Input: dimensioned drawing with shaded views. Units: mm. Origin: part minimum x, y, z. Round coordinates to 2 decimals unless told otherwise and drop trailing zeros. Write each loop counter-clockwise with the first axis right and the second up, starting at its lowest first coordinate (ties: lowest second). Pieces come first, ordered by that corner, then holes. Notation, with made-up numbers: (-1.5, 34) -> (19.5, 34) arc R20 ccw to (19.5, 52) -> close; hole circle Ø5 at (5.5, 41.5). An arc over 180 degrees is marked (long way). Use one line per item in the form item = value. Start each with the question number.
1. Cut plane B-B, the plane x = 60. Return the cut outline in (y, z).
2. Draft query along Y for the marked faces 1, 2, 3 and 4. Return one class per face: pulls with the +Y half, pulls with the -Y half, needs draft (parallel to the pull), parting line crosses it, or undercut.
3. Pin query (flat end, axial travel): pin 1 Ø5 at (x, y) = (55.5, 28) entering from +Z; pin 2 Ø2 at (x, y) = (79, 19.5) entering from -Z; pin 3 Ø3 at (y, z) = (50, 2) entering from -X (3 decimals). Return the tip coordinate at first contact, or that it passes through.
4. Cut plane D-D, the plane z = 4.5. Return the cut outline in (x, y) (3 decimals).
5. Line query: L1, parallel to Y at x = 31.5, z = 8.75; L2, parallel to X at y = 44.5, z = 13.5; L3, parallel to Z at x = 5, y = 54. Output: solid intervals per line, ascending.
6. Cut plane C-C, the plane y = 48. Return the cut outline in (x, z), plus the area to 3 significant figures.
7. Cut plane A-A, the plane z = 12. Return the cut outline in (x, y), plus the area to 3 significant figures.
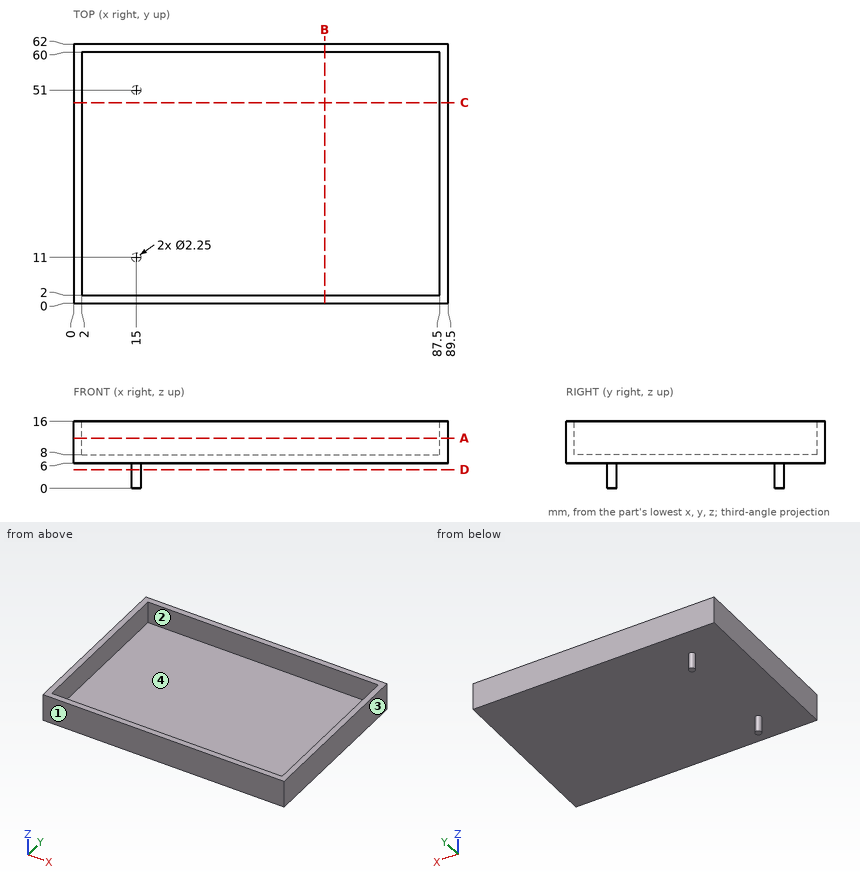
Outcome:
q1.outline = (0, 6) -> (62, 6) -> (62, 16) -> (60, 16) -> (60, 8) -> (2, 8) -> (2, 16) -> (0, 16) -> close
q2.face_1 = pulls with the -Y half
q2.face_2 = undercut
q2.face_3 = needs draft
q2.face_4 = undercut
q3.pin_1 = 8
q3.pin_2 = 6
q3.pin_3 = 13.875
q4.outline = circle Ø2.25 at (15, 11); circle Ø2.25 at (15, 51)
q5.L1 = 0 to 2, 60 to 62
q5.L2 = 0 to 2, 87.5 to 89.5
q5.L3 = 6 to 8
q6.outline = (0, 6) -> (89.5, 6) -> (89.5, 16) -> (87.5, 16) -> (87.5, 8) -> (2, 8) -> (2, 16) -> (0, 16) -> close
q6.area = 211 mm^2
q7.outline = (0, 0) -> (89.5, 0) -> (89.5, 62) -> (0, 62) -> close; hole (2, 2) -> (87.5, 2) -> (87.5, 60) -> (2, 60) -> close
q7.area = 590 mm^2
